The listing builds one solid part. Answer for the finished solid, in the listing's coordinates (mm). A direction names the side the tool comes from. Round coordinates to 2 decimals unless told otherwise and drop trailing zeros. Order: outer loops, then holes, each group sorted by start corner. A loop starts at its lowest first (then second) coordinate and runs counter-clockwise, first axis right, second up. Notation, with made-up numbers: (88, -9.5) - (134, -9.5) arc R25 ccw to (134, 24.5) - close; hole circle Ø8 at (16.5, -16). An arc over 180 degrees is marked (long way). Use CSV: the item, a comma, the result in double quotes. Start each with the question number.
Item 1: For faces 1 (the flat face through (6, -4, -4)), 2 (the flat face through (3, 16, 3.397)), determine the directions among +Z, -Z, +X, -X, +Y, -Y from which every point of the face is accessible in a straight line to the end or side of a thin tool.
Item 2: Find section D-D, the plane y = -13. Give the vertices of the cut face in (x, z), plus the area to 3 significant figures.
Item 3: Flat-ended cylindrical pins translate along their axes: P1, Ø1, axis at x = 2, z = 12.5, coming from the -Y side; P2, Ø2, axis at x = 1.5, y = 16.5, coming from the +Z side; P3, Ø3, axis at x = 1, z = -9.5, coming from the -Y side; P4, Ø3, axis at y = 0, z = 14, coming from the -X side (1 decimal). Find the tip coordinate at first contact, or state that the pin passes through.
Item 4: Determine the mould class of faces 3 (the cylindrical face through (3, 0.1, 16.5)), 4 (the cylindrical face through (2.958, 17.374, -0.028)), 5 (the flat face through (0, -4, -4)) for opening direction Z: +Z half, -Z half, draft (parallel to the pull), parting line (faces both ways), or undercut.
Item 5: Find section B-B, the plane y = -3. Give the vertices of the cut face in (x, z), plus the area to 3 significant figures.
Item 6: Find section A-A, the plane z = 0. Give the vertices of the cut face in (x, y), plus the area to 3 significant figures.
Item 7: Straight lines are drawn through the part: line 1 along Y through (x, z) = (1.5, 0); line 2 along Z through (x, y) = (0.5, -2); line 3 along Z through (x, y) = (3.7, -3.5). For each, find the intervals that lie inside material, in ascending order. Write a range as [from, to].
Item 8: Find section C-C, the plane x = 0.9. Give the vertices of the cut face in (y, z).
```python
from build123d import *

# Parameters (mm, degrees)
SKETCH1_R           = 2.5
SKETCH1_R_2         = 5.9055
BOSS_EXTRUDE1_DEPTH = 6


with BuildPart() as part:
    # Sketch1 → Boss-Extrude1 (new body)
    with BuildSketch(Plane(origin=(0, 0, 0), x_dir=(0, 0, -1), z_dir=(1, 0, 0))):
        with BuildLine():
            ThreePointArc((3.397, 14.755273557), (2.6985, 14.056773557), (2, 14.755273557))
            Line((2, 14.755273557), (2, 17.25809888))
            ThreePointArc((2, 17.25809888), (0, 17.3736), (-2, 17.25809888))
            Line((-2, 17.25809888), (-2, 14.755273557))
            ThreePointArc((-2, 14.755273557), (-2.6985, 14.056773557), (-3.397, 14.755273557))
            Line((-3.397, 14.755273557), (-3.397, 17.038261882))
            ThreePointArc((-3.397, 17.038261882), (-11.018708131, -13.432425249), (17.3736, 0))
            ThreePointArc((17.3736, 0), (13.432425249, 11.018708131), (3.397, 17.038261882))
            Line((3.397, 17.038261882), (3.397, 14.755273557))
        make_face()
        with Locations((-14, 0)):
            Circle(SKETCH1_R, mode=Mode.SUBTRACT)
        with Locations((14, 0)):
            Circle(SKETCH1_R, mode=Mode.SUBTRACT)
        with Locations((0, 1.3715)):
            Circle(SKETCH1_R_2, mode=Mode.SUBTRACT)
    extrude(amount=BOSS_EXTRUDE1_DEPTH)


solid = part.part
```
Worked out:
1,face 1,"+Z, -Z, +X, +Y, -Y"
1,face 2,"+X, -X, +Y"
2,outline,"(0, -11.53) - (6, -11.53) - (6, 11.53) - (0, 11.53) - close"
2,area,"138 mm²"
3,P1,"stops at y = -12.56"
3,P2,"stops at z = 7.85"
3,P3,"stops at y = -15.42"
3,P4,"passes through"
4,face 3,"undercut"
4,face 4,"parting line"
4,face 5,"draft"
5,outline,"(0, -17.11) - (6, -17.11) - (6, -3.97) - (0, -3.97) - close; (0, 3.97) - (6, 3.97) - (6, 17.11) - (0, 17.11) - close"
5,area,"158 mm²"
6,outline,"(0, -17.37) - (6, -17.37) - (6, -4.53) - (0, -4.53) - close; (0, 7.28) - (6, 7.28) - (6, 17.37) - (0, 17.37) - close"
6,area,"138 mm²"
7,line 1,"y = [-17.37, -4.53], [7.28, 17.37]"
7,line 2,"z = [-17.26, -15.5], [-12.5, -4.85], [4.85, 12.5], [15.5, 17.26]"
7,line 3,"z = [-17.02, -3.34], [3.34, 17.02]"
8,outline,"(14.76, -3.4) arc R0.7 cw to (14.76, -2) - (17.26, -2) arc R17.37 ccw to (17.26, 2) - (14.76, 2) arc R0.7 cw to (14.76, 3.4) - (17.04, 3.4) arc R17.37 ccw (long way) to (17.04, -3.4) - close; hole circle Ø11.81 at (1.37, 0); hole circle Ø5 at (0, -14); hole circle Ø5 at (0, 14)"
